The figure shows three views and two pictorial views of one solid part (mm, origin at its lowest corner). Answer the questions. Round coordinates to 2 decimals unless told otherwise and drop trailing zeros. Order: outer loops, then holes, each group sorted by start corner. A loop starts at its lowest first (then second) coordinate and runs counter-clockwise, first axis right, second up. Notation, with made-up numbers: (87.25, 79) -> (104.25, 79) arc R11 cw to (104.25, 96) -> close; hole circle Ø4 at (-15, 51). An arc over 180 degrees is marked (long way). Return JSON: item names as keys, results as strings. Group by question number.
(1) The part is cut by section B-B (x = 78.5). Determine the outline of the cut face in (y, z).
(2) The part is cut by section A-A (z = 66.04). Determine the outline of the cut face in (x, y), plus the area to 3 significant figures.
(3) Consider line 1 (Z direction, x = 46, y = 3.5); line 2 (X direction, y = 4, z = 53); line 3 (X direction, y = 3.5, z = 66.04). Determine where each line is inside the solid, lowest interval first. Write a range as [from, to].
(4) The part is cut by section C-C (y = 3.5). Determine the outline of the cut face in (x, z).
(5) Each of these flat-tipped pins is pushed along its axis until it touches: pin 1 (8 mm diameter, centred on x = 88, z = 16.5, fed in from -Y); pin 2 (2 mm diameter, centred on y = 5, z = 99, fed in from +X); pin 3 (1.5 mm diameter, centred on x = 25, y = 2.5, fed in from +Z); pin 4 (6 mm diameter, centred on x = 104.14, z = 76.2, fed in from -Y). Where does it stop, or does it pass through?
(6) The part is cut by section D-D (z = 25). Determine the outline of the cut face in (x, y), plus the area to 3 significant figures.
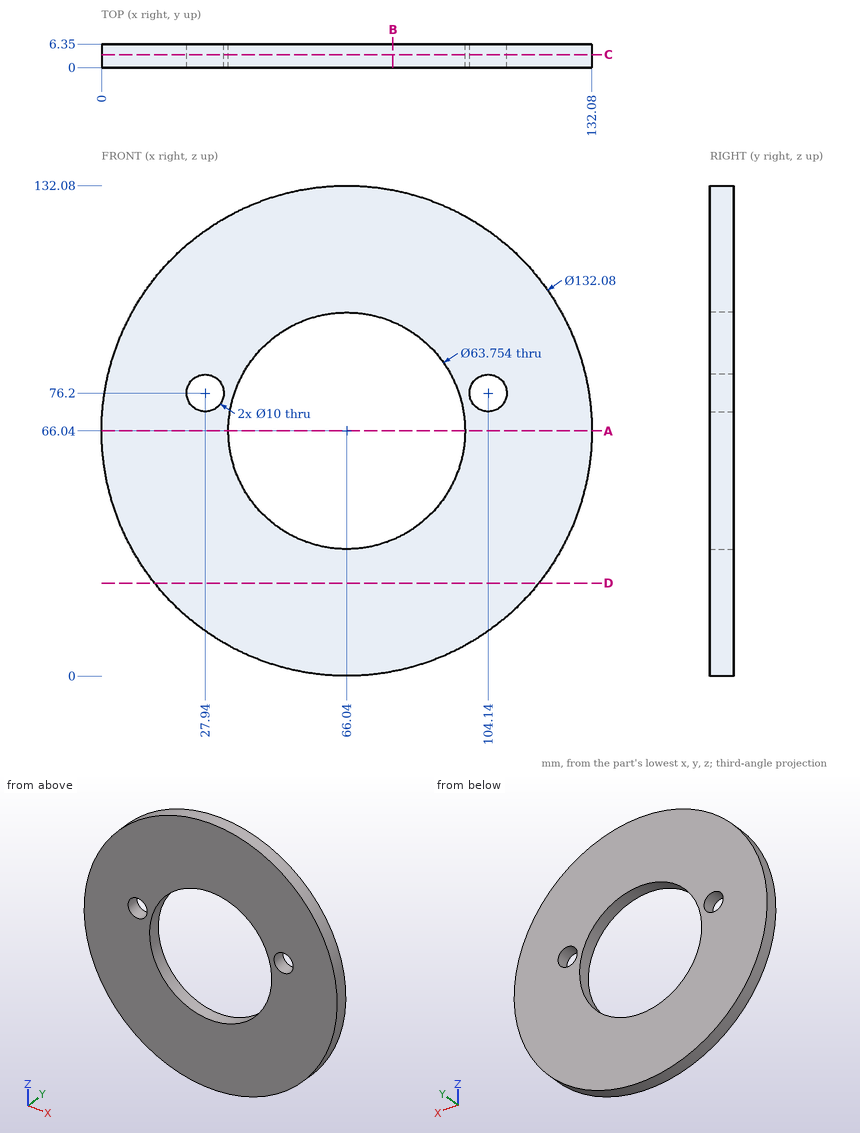
Answer below:
{
 "1": {"outline": "(0, 1.19) -> (6.35, 1.19) -> (6.35, 36.7) -> (0, 36.7) -> close; (0, 95.38) -> (6.35, 95.38) -> (6.35, 130.89) -> (0, 130.89) -> close"},
 "2": {"outline": "(0, 0) -> (34.16, 0) -> (34.16, 6.35) -> (0, 6.35) -> close; (97.92, 0) -> (132.08, 0) -> (132.08, 6.35) -> (97.92, 6.35) -> close", "area": "434 mm²"},
 "3": {"line 1": "z = [3.11, 41.25], [90.83, 128.97]", "line 2": "x = [1.3, 36.95], [95.13, 130.78]", "line 3": "x = [0, 34.16], [97.92, 132.08]"},
 "4": {"outline": "circle Ø132.08 at (66.04, 66.04); hole circle Ø10 at (27.94, 76.2); hole circle Ø63.75 at (66.04, 66.04); hole circle Ø10 at (104.14, 76.2)"},
 "5": {"pin 1": "stops at y = 0", "pin 2": "stops at x = 123.83", "pin 3": "stops at z = 118.37", "pin 4": "passes through"},
 "6": {"outline": "(14.3, 0) -> (117.78, 0) -> (117.78, 6.35) -> (14.3, 6.35) -> close", "area": "657 mm²"}
}
